```python
from build123d import *

# Parameters (mm, degrees)
F0_W     = 20
F0_H     = 40
F0_H_2   = 35
F1_DEPTH = 20


with BuildPart() as f1:
    # F0 (on Front) → F1 (new body)
    with BuildSketch(Plane.XZ):
        Polygon((118.989712, 78.679), (-211.010288, 78.679), (-211.010288, -71.321), (118.989712, -71.321), (118.989712, -31.321), (118.989712, 3.679), (118.989712, 38.679), align=None)
        with Locations((128.989712, 58.679)):
            Rectangle(F0_W, F0_H)
        with Locations((128.989712, -13.821)):
            Rectangle(F0_W, F0_H_2)
    extrude(amount=F1_DEPTH)


solid = f1.part
```
Work out the finished part from the listing and answer in its coordinate system (mm). A direction names the side the tool comes from. Give positions to 0.01 mm unless a question says otherwise; leave off trailing zeros. Order: outer loops, then holes, each group sorted by start corner. A loop starts at its lowest first (then second) coordinate and runs counter-clockwise, first axis right, second up. Notation, with made-up numbers: (31.5, 43.5) - (39.5, 43.5) arc R20 cw to (39.5, 81.5) - close; hole circle Ø6 at (-20, -27.5). An arc over 180 degrees is marked (long way). One line per item, written item: value. Start each with the question number.
1. Which of the six approach directions +Z, -Z, +X, -X, +Y, -Y give full straight-line access (tool end or side, diameter ignored) to faces 1 (the face through (129, -10, 38.679)), 2 (the face through (-38, 0, 5)), 3 (the face through (118.99, -10, -52))?
2. For a pull along Z with two mould halves and no side action, classify faces 4 (the face through (138.99, -10, 58)), 5 (the face through (-34, -10, 78.679)), 6 (the face through (118.99, -10, 21)) as released by +Z, released by -Z, zero draft, split by the parting line, or undercut.
3. Section B-B, the plane z = 26 is taken. Write down the section's boundary in (x, y), then the cut area to 3 significant figures.
4. Each of these flat-tipped pins is pushed along its axis until it touches: pin 1 Ø8 at (x, z) = (-26.5, 41.5) entering from +Y; pin 2 Ø10 at (y, z) = (-8, -41.5) entering from +X; pin 3 Ø10 at (x, y) = (128.5, -12.5) entering from -Z. Where does it stop, or does it pass through?
5. Section A-A, the plane y = -8 is taken. Write down the section's boundary in (x, z).
6. Consider line 1 (X direction, y = -13.5, z = 7). Determine where the line is inside the solid, lowest interval first.
Filled sheet:
1. face 1: +X, +Y, -Y
1. face 2: +Z, -Z, +X, -X, +Y
1. face 3: -Z, +X, +Y, -Y
2. face 4: zero draft
2. face 5: released by +Z
2. face 6: undercut
3. outline: (-211.01, -20) - (118.99, -20) - (118.99, 0) - (-211.01, 0) - close
3. area: 6,600 mm²
4. pin 1: y = 0
4. pin 2: x = 118.99
4. pin 3: z = -31.32
5. outline: (-211.01, -71.32) - (118.99, -71.32) - (118.99, -31.32) - (138.99, -31.32) - (138.99, 3.68) - (118.99, 3.68) - (118.99, 38.68) - (138.99, 38.68) - (138.99, 78.68) - (-211.01, 78.68) - close
6. line 1: -211.01 to 118.99
